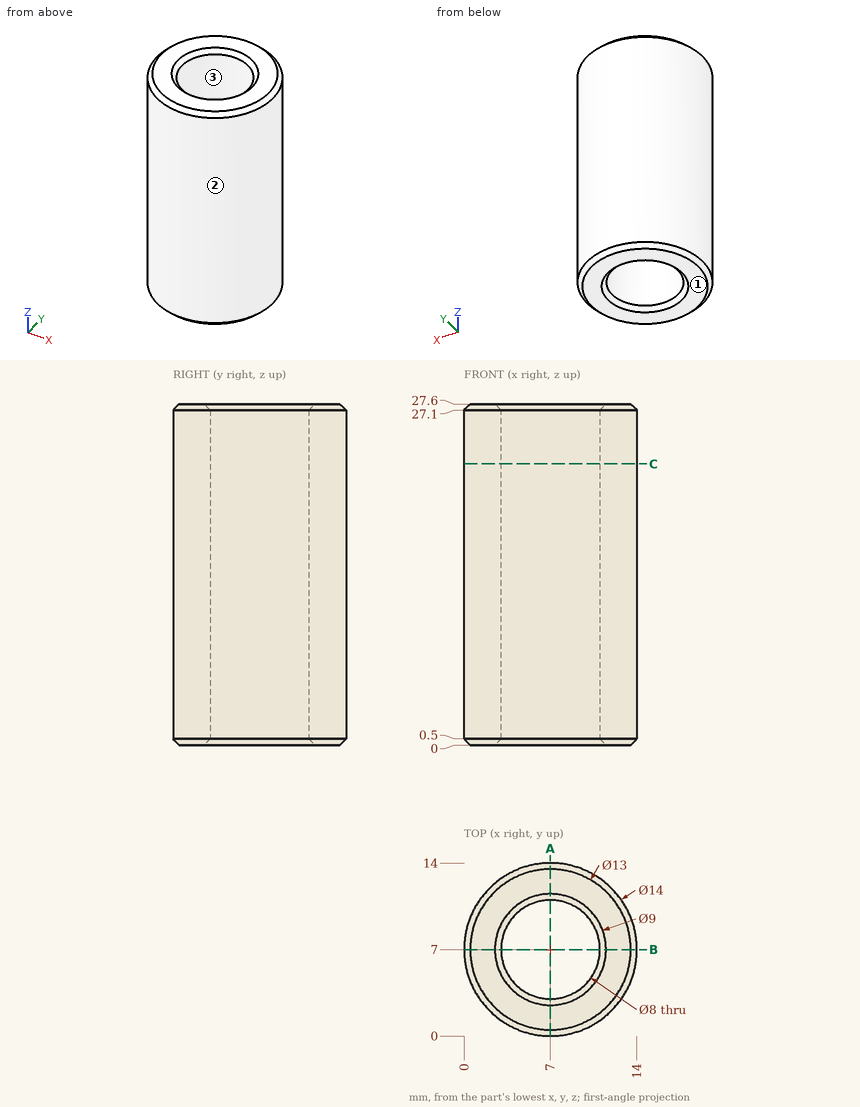
The figure shows three views and two pictorial views of one solid part (mm, origin at its lowest corner). Answer the questions. Give positions to 0.01 mm unless a question says otherwise; leave off trailing zeros. Write each loop counter-clockwise with the first axis right and the second up, starting at its lowest first coordinate (ties: lowest second). Pieces come first, ordered by that corner, then holes. Notation, with made-up numbers: (81, -16.5) - (102, -16.5) arc R7 cw to (102, -9.5) - close; hole circle Ø2 at (-1.5, -26.5). An arc over 180 degrees is marked (long way). Use CSV: the item, a comma, the result in double quotes. Start each with the question number.
Item 1: The mould has two halves that part along X. Classify the marked faces 1, 2 and 3: pulls with the +X half, pulls with the -X half, needs draft (parallel to the pull), parting line crosses it, or undercut.
Item 2: The part is cut by section A-A, the plane x = 7. Give the vertices of the cut face in (y, z).
Item 3: Consider line 1 (Y direction, x = 7, z = 13.25); line 2 (Y direction, x = 3.75, z = 17.5); line 3 (X direction, y = 4.75, z = 23.75). Determine where each line is inside the solid, lowest interval first.
Item 4: The part is cut by section C-C, the plane z = 22.75. Give the vertices of the cut face in (x, y), and give its area (3 significant figures).
Item 5: Flat-ended cylindrical pins translate along their axes: P1, Ø1.5, axis at y = 10, z = 20, coming from the -X side; P2, Ø1.5, axis at x = 2.5, z = 15.5, coming from the +Y side; P3, Ø2, axis at x = 8.5, z = 7.5, coming from the +Y side. Find the tip coordinate at first contact, or state that the pin passes through.
Taken from the geometry:
1,face 1,"needs draft"
1,face 2,"parting line crosses it"
1,face 3,"undercut"
2,outline,"(0, 0.5) - (0.5, 0) - (2.5, 0) - (3, 0.5) - (3, 27.1) - (2.5, 27.6) - (0.5, 27.6) - (0, 27.1) - close; (11, 0.5) - (11.5, 0) - (13.5, 0) - (14, 0.5) - (14, 27.1) - (13.5, 27.6) - (11.5, 27.6) - (11, 27.1) - close"
3,line 1,"0 to 3, 11 to 14"
3,line 2,"0.8 to 4.67, 9.33 to 13.2"
3,line 3,"0.37 to 3.69, 10.31 to 13.63"
4,outline,"circle Ø14 at (7, 7); hole circle Ø8 at (7, 7)"
4,area,"104 mm2"
5,P1,"x = 0.37"
5,P2,"y = 12.91"
5,P3,"y = 13.98"
